```python
from build123d import *

# Parameters (mm, degrees)
SKETCH5_R                = 3.51
SKETCH5_R_2              = 2
BOSS_EXTRUDE1_DEPTH      = 3
BOSS_EXTRUDE1_DEPTH_BACK = 3
BOSS_EXTRUDE2_START      = -3
SKETCH7_R                = 5
SKETCH7_R_2              = 3.51
BOSS_EXTRUDE2_DEPTH      = 1.5


with BuildPart() as part:
    # Sketch5 → Boss-Extrude1 (new body, two sides)
    with BuildSketch(Plane(origin=(0, 0, 0), x_dir=(1, 0, 0), z_dir=(0, 1, 0))) as boss_extrude1_sk:
        Circle(SKETCH5_R)
        Circle(SKETCH5_R_2, mode=Mode.SUBTRACT)
    extrude(amount=BOSS_EXTRUDE1_DEPTH)
    extrude(boss_extrude1_sk.sketch, amount=-BOSS_EXTRUDE1_DEPTH_BACK)

    # Sketch7 → Boss-Extrude2 (add)
    with BuildSketch(Plane(origin=(0, 0, 0), x_dir=(1, 0, 0), z_dir=(0, 1, 0)).offset(BOSS_EXTRUDE2_START)):
        Circle(SKETCH7_R)
        Circle(SKETCH7_R_2, mode=Mode.SUBTRACT)
    extrude(amount=BOSS_EXTRUDE2_DEPTH)


solid = part.part
```
Source: CAD feature listing. Evaluate the final solid. Frame: model axes, mm. A direction names the side the tool comes from. Give positions to 0.01 mm unless a question says otherwise; leave off trailing zeros. Loops run counter-clockwise (first coordinate to the right, second up) from the corner with the lowest first, then second, coordinate; pieces in that order, holes last. Notation, with made-up numbers: (-3, 39.5) -> (8, 39.5) arc R26 cw to (8, 63.5) -> close; hole circle Ø7 at (-10, 42). An arc over 180 degrees is marked (long way). Put each result on its own line as item: value. Start each with the question number.
1) Material intervals for probe 1 along Z at (x, y) = (0, 1.7); probe 2 along X at (y, z) = (-1.55, 0), sorted ascending.
2) Contact query for flat-ended pins moving along their axis: P1, Ø1, axis at x = -2, y = 1.5, coming from the -Z side; P2, Ø3, axis at x = 0, z = 0, coming from the +Y side; P3, Ø6, axis at x = 3, z = -2, coming from the +Y side; P4, Ø3, axis at y = 0.5, z = 2.5, coming from the -X side. Output: stop coordinate, or through.
3) Reachability of faces 1 (the face through (-1.08, -2.26, 4.88)), 2 (the face through (2.2, -1.5, 3.3)) from +Z, -Z, +X, -X, +Y, -Y: full face, straight path, thin tool, end or side. Return the list, or none.
4) Cut plane A-A (z = 0). Return loops of the section in (x, y), then the cut area to 3 significant figures.
5) Cut plane B-B (x = 0). Return loops of the section in (y, z).
6) Cut plane C-C (x = 2.75). Return loops of the section in (y, z).
7) Cut plane D-D (y = -0.7). Return loops of the section in (x, z).
Results are:
1. probe 1: z = -3.51 to -2, 2 to 3.51
1. probe 2: x = -5 to -2, 2 to 5
2. P1: stops at z = -3.17
2. P2: passes through
2. P3: stops at y = 3
2. P4: stops at x = -3.36
3. face 1: +Y, -Y
3. face 2: +Y
4. outline: (-5, -3) -> (-2, -3) -> (-2, 3) -> (-3.51, 3) -> (-3.51, -1.5) -> (-5, -1.5) -> close; (2, -3) -> (5, -3) -> (5, -1.5) -> (3.51, -1.5) -> (3.51, 3) -> (2, 3) -> close
4. area: 22.6 mm2
5. outline: (-3, -5) -> (-1.5, -5) -> (-1.5, -3.51) -> (3, -3.51) -> (3, -2) -> (-3, -2) -> close; (-3, 2) -> (3, 2) -> (3, 3.51) -> (-1.5, 3.51) -> (-1.5, 5) -> (-3, 5) -> close
6. outline: (-3, -4.18) -> (-1.5, -4.18) -> (-1.5, -2.18) -> (3, -2.18) -> (3, 2.18) -> (-1.5, 2.18) -> (-1.5, 4.18) -> (-3, 4.18) -> close
7. outline: circle Ø7.02 at (0, 0); hole circle Ø4 at (0, 0)
